from build123d import *

# Parameters (mm, degrees)
F0_W     = 101.6
F0_H     = 38.1
F1_DEPTH = 19.05
F2_R     = 3.175
F4_D     = 3.175


with BuildPart() as f1:
    # F0 (on Top) → F1 (new body)
    with BuildSketch(Plane.XY):
        Rectangle(F0_W, F0_H)
    extrude(amount=F1_DEPTH)

    # F2
    f2_edges = [f1.edges().sort_by_distance(p)[0] for p in [
        (-50.8, 19.05, 9.525),
        (-50.8, -19.05, 9.525),
        (50.8, 19.05, 9.525),
        (50.8, -19.05, 9.525),
    ]]
    fillet(f2_edges, radius=F2_R)

    # F4 (through all)
    with Locations(Plane.XY.offset(19.05)):
        with Locations((-47.625, 0), (47.625, 0)):
            Hole(F4_D / 2)


solid = f1.part
Check sheet for the modelled part. Datum: model origin and axes. Units: mm. Give positions to 0.01 mm unless a question says otherwise; leave off trailing zeros. Write each loop counter-clockwise with the first axis right and the second up, starting at its lowest first coordinate (ties: lowest second). Pieces come first, ordered by that corner, then holes. Notation, with made-up numbers: (-10, -16.75) -> (43, -16.75) arc R28 cw to (43, 12.25) -> close; hole circle Ø7 at (26, 53.25). An arc over 180 degrees is marked (long way). One line per item, written item: value. Start each with the question number.
Item 1: Draft check along Y on faces 1 (the cylindrical face through (-49.89, -18.1, 9.66)), 2 (the cylindrical face through (-49.14, 0.48, 9.39)), 3 (the cylindrical face through (49.89, 18.1, 9.66)). Enter one of: +Y half, -Y half, draft (parallel to the pull), parting line (faces both ways), or undercut.
Item 2: Material ranges on probe 1 along X at (y, z) = (-1, 16.75); probe 2 along X at (y, z) = (16.5, 6.5), recorded low to high. Write a range as from..to.
Item 3: Section check A-A on y = 0. Record the cut outline in (x, z), then the cut area to 3 significant figures.
Results list:
1. face 1: -Y half
1. face 2: undercut
1. face 3: +Y half
2. probe 1: -50.8..-48.86, -46.39..46.39, 48.86..50.8
2. probe 2: -50.74..50.74
3. outline: (-50.8, 0) -> (-49.21, 0) -> (-49.21, 19.05) -> (-50.8, 19.05) -> close; (-46.04, 0) -> (46.04, 0) -> (46.04, 19.05) -> (-46.04, 19.05) -> close; (49.21, 0) -> (50.8, 0) -> (50.8, 19.05) -> (49.21, 19.05) -> close
3. area: 1,810 mm²
